Check sheet for the drawn part. Datum: minimum x, y, z corner. Units: mm. Round coordinates to 2 decimals unless told otherwise and drop trailing zeros. Write each loop counter-clockwise with the first axis right and the second up, starting at its lowest first coordinate (ties: lowest second). Pieces come first, ordered by that corner, then holes. Notation, with made-up numbers: M 11,48 L 50,48 A15 cw 50,74 Z; hole C 79,23.5 d7. An arc over 180 degrees is marked long. One line per item, written item: value. Start each with the question number.
1. Release check for a two-part mould opening along Y. For the marked faces 1, 2, 3 and 4 record: pulls with the +Y half, pulls with the -Y half, needs draft (parallel to the pull), parting line crosses it, or undercut.
2. Scan lines: probe 1 along X at (y, z) = (4.5, 4.75); probe 2 along X at (y, z) = (8, 1.75) (1 decimal); probe 3 along Y at (x, z) = (5.5, 0.75) (1 decimal). Record each from-to range of solid material in increasing order. Write a range as [from, to].
3. Section check A-A (z = 2.5). Record the boundary of the cut face in (x, y) (1 decimal).
4. Depth check by flat-ended pin: P1, Ø1.5, axis at x = 2.5, z = 3, coming from the -Y side; P2, Ø3, axis at y = 6.5, z = 3, coming from the -X side (1 decimal); P3, Ø1.5, axis at y = 7, z = 1.5, coming from the -X side; P4, Ø1.8, axis at x = 4.445, y = 4.445, coming from the +Z side. Enter the tip coordinate at first touch or a pass-through.
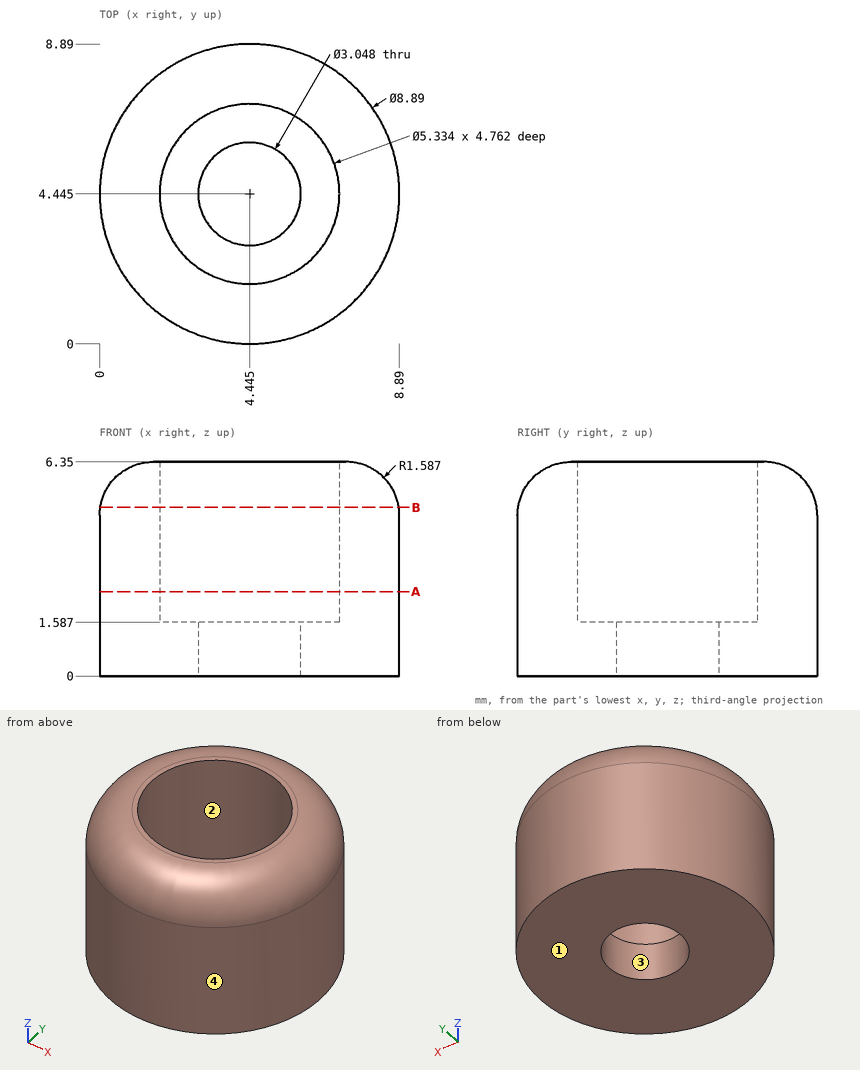
Result sheet:
1. face 1: needs draft
1. face 2: undercut
1. face 3: undercut
1. face 4: parting line crosses it
2. probe 1: x = [0, 1.78], [7.11, 8.89]
2. probe 2: x = [1.8, 7.1]
2. probe 3: y = [0.1, 3.3], [5.5, 8.8]
3. outline: C 4.4,4.4 d8.9; hole C 4.4,4.4 d5.3
4. P1: stops at y = 0.16
4. P2: stops at x = 0
4. P3: stops at x = 0.38
4. P4: passes through
